Autodesk Fusion 360 part; units mm, degrees
sketch "Sketch1" plane through (0, 0, 0) normal (0, 1, 0) x (1, 0, 0)
  line L0 (0, 0) -> (78, 0)
  line L1 (0, 0) -> (0, -43)
  line L2 (0, -43) -> (78, -43)
  line L3 (78, 0) -> (78, -43)
  line L4 (0, 5) -> (83, 5)
  line L5 (83, 5) -> (83, -48)
  line L6 (83, -48) -> (-5, -48)
  line L7 (-5, -48) -> (-5, 5)
  line L8 (-5, 5) -> (0, 5)
  dimension "d1" = 78
  dimension "d2" = 43
  dimension "d3" = 78
  dimension "d4" = 5
  dimension "d5" = 83
  dimension "d6" = 53
  dimension "d7" = 88
extrude "Extrude1" add sketch "Sketch1" along normal blind 23
sketch "Sketch2" plane through (0, 0, 0) normal (0, 1, 0) x (1, 0, 0)
sketch "Sketch3" plane through (0, 0, 0) normal (0, 1, 0) x (1, 0, 0)
  line L0 (0, 0) -> (78, 0)
  line L1 (78, 0) -> (78, -43)
  line L2 (78, -43) -> (0, -43)
  line L3 (0, -43) -> (0, 0)
extrude "Extrude2" add sketch "Sketch3" along normal blind 3
sketch "Sketch4" plane through (0, 3, 0) normal (0, 1, 0) x (-1, 0, 0)
  line L0 (0, 43) -> (-78, 43)
  line L1 (-78, 43) -> (-78, 0)
  line L2 (-78, 0) -> (0, 0)
sketch "Sketch5" plane through (0, 0, 0) normal (0, -1, 0) x (1, 0, 0)
  line L0 (-5, 48) -> (-5, -5)
  line L1 (-5, -5) -> (83, -5)
  line L2 (83, -5) -> (83, 48)
  line L3 (83, 48) -> (-5, 48)
sketch "Sketch6" plane through (0, 3, 0) normal (0, 1, 0) x (-1, 0, 0)
  line L0 (-39, 21.5) -> (-39, 11.75)
  line L1 (-39, 21.5) -> (-39, 31.25)
  circle A0 centre (-39, 11.75) radius 1.75
  circle A1 centre (-39, 31.25) radius 1.75
  dimension "d12" = 9.75
  dimension "d13" = 9.75
  dimension "d14" = 3.5
  dimension "d15" = 3.5
extrude "Extrude3" cut sketch "Sketch6" against normal blind 20
sketch "Sketch7" plane through (0, 3, 0) normal (0, 1, 0) x (-1, 0, 0)
  circle A0 centre (-39, 11.75) radius 1.75
  circle A1 centre (-39, 31.25) radius 1.75
  line L0 (0, 43) -> (-78, 43)
  line L1 (-78, 0) -> (0, 0)
  line L2 (0, 0) -> (0, 43)
sketch "Sketch8" plane through (0, 3, 0) normal (0, 1, 0) x (-1, 0, 0)
sketch "Sketch9" plane through (83, 0, 0) normal (1, 0, 0) x (0, 0, -1)
  line L0 (-48, 0) -> (5, 0)
  line L1 (5, 0) -> (5, 23)
  line L2 (5, 23) -> (-48, 23)
  line L3 (-48, 23) -> (-48, 0)
sketch "Sketch10" plane through (83, 0, 0) normal (1, 0, 0) x (0, 0, -1)
  line L0 (-48, 0) -> (-48, 3)
  line L1 (5, 3) -> (-21.5, 3)
  line L2 (-21.5, 3) -> (-24.5, 3)
  arc A0 (-18.5, 3) -> (-24.5, 3) centre (-21.5, 3) ccw
  dimension "d18" = 3
  dimension "d19" = 6
extrude "Extrude4" cut sketch "Sketch10" against normal blind 20
sketch "Sketch11" plane through (83, 0, 0) normal (1, 0, 0) x (0, 0, -1)
  line L0 (-21.5, 3) -> (-21.5, 6)
  line L1 (-21.5, 6) -> (-21.5, 23)
  line L2 (-21.5, 23) -> (-21.5, 14.5)
  circle A0 centre (-40, 14.5) radius 2.5
  line L3 (-21.5, 14.5) -> (-3, 14.5)
  circle A1 centre (-3, 14.5) radius 2.5
  dimension "d22" = 5
  dimension "d24" = 18.5
  dimension "d25" = 5
extrude "Extrude5" cut sketch "Sketch11" against normal blind 50
sketch "Sketch12" plane through (0, 0, -5) normal (0, 0, -1) x (-1, 0, 0)
  line L0 (-83, 0) -> (5, 0)
  line L1 (5, 0) -> (5, 23)
  line L2 (5, 23) -> (-83, 23)
  line L3 (-83, 23) -> (-83, 0)
  line L4 (-39, 20) -> (-50, 20)
  line L5 (-50, 20) -> (-50, 17)
  line L6 (-50, 17) -> (-28, 17)
  line L7 (-28, 17) -> (-28, 20)
  line L8 (-28, 20) -> (-39, 20)
  dimension "d29" = 3
  dimension "d30" = 22
extrude "Extrude6" cut sketch "Sketch12" against normal blind 100 contours L4 L5 L6 L7 L8
Build history of the part. All positions in model axes, mm. A direction names the side the tool comes from. Round coordinates to 2 decimals unless told otherwise and drop trailing zeros. Write each loop counter-clockwise with the first axis right and the second up, starting at its lowest first coordinate (ties: lowest second). Pieces come first, ordered by that corner, then holes. Notation, with made-up numbers: (-25.75, 44.5) -> (13.25, 44.5) arc R14 ccw to (13.25, 70.5) -> close; hole circle Ø1 at (18.25, 72.5). An arc over 180 degrees is marked (long way). Put each result on its own line as item: value.
Item 1: Two-plate mould, pull along Z, no slides. Class faces 5 (the face through (50, 19, 45)), 6 (the face through (37.383, 1.521, 11.08)), 7 (the face through (40, 11, 48)): pulls with the +Z half, pulls with the -Z half, needs draft (parallel to the pull), parting line crosses it, or undercut.
Here are the results:
face 5: needs draft
face 6: undercut
face 7: pulls with the +Z half
Item 2: Wall check: probe 1 along Z at (x, y) = (39, 0.8); probe 2 along Z at (x, y) = (20.5, 15); probe 3 along X at (y, z) = (10, 11). Give the ranges that are in metal, low to high. Write a range as from..to.
Here are the results:
probe 1: z = -5..10, 13.5..29.5, 33..48
probe 2: z = -5..0, 43..48
probe 3: x = -5..0, 78..83
Item 3: Slice it at D-D, the plane y = 7.5. Give the cut face in (x, z).
Here are the results:
outline: (-5, -5) -> (83, -5) -> (83, 48) -> (-5, 48) -> close; hole (0, 0) -> (78, 0) -> (78, 43) -> (0, 43) -> close
Item 4: Flat gauge pin, fed straight in: P1, Ø4, axis at x = 39, z = 31.25, coming from the +Y side. Where does the tip first touch, or does it go through?
Here are the results:
P1: stops at y = 3
Item 5: Tool access for faces 1 (the face through (78, 13, 21)), 2 (the face through (83, 11, 21)), 3 (the face through (28, 18, -3)), 4 (the face through (80.54, 13.54, 37.69)): list every direction of +Z, -Z, +X, -X, +Y, -Y with a clear straight run to the whole face (end or side of a thin tool).
Here are the results:
face 1: +Y
face 2: +Z, -Z, +X, +Y, -Y
face 3: +Z, -Z
face 4: +X
Item 6: Slice it at C-C, the plane z = 21.5. Give the cut face in (x, y).
Here are the results:
outline: (-5, 0) -> (83, 0) -> (83, 3) -> (0, 3) -> (0, 23) -> (-5, 23) -> close; (78, 6) -> (83, 6) -> (83, 23) -> (78, 23) -> close
Item 7: Slice it at A-A, the plane y = 13. Give the cut face in (x, z).
Here are the results:
outline: (-5, -5) -> (83, -5) -> (83, 1) -> (78, 1) -> (78, 0) -> (0, 0) -> (0, 43) -> (78, 43) -> (78, 42) -> (83, 42) -> (83, 48) -> (-5, 48) -> close; (78, 5) -> (83, 5) -> (83, 38) -> (78, 38) -> close
Item 8: Slice it at B-B, the plane x = 39. Give the cut face in (y, z).
Here are the results:
outline: (0, -5) -> (17, -5) -> (17, 0) -> (3, 0) -> (3, 10) -> (0, 10) -> close; (0, 13.5) -> (3, 13.5) -> (3, 29.5) -> (0, 29.5) -> close; (0, 33) -> (3, 33) -> (3, 43) -> (17, 43) -> (17, 48) -> (0, 48) -> close; (20, -5) -> (23, -5) -> (23, 0) -> (20, 0) -> close; (20, 43) -> (23, 43) -> (23, 48) -> (20, 48) -> close
